```python
from build123d import *

# Parameters (mm, degrees)
SKETCH_1_W          = 206
SKETCH_1_H          = 36
SKETCH_1_W_2        = 200
SKETCH_1_H_2        = 30
EXTRUDE_1_DEPTH     = 20
SKETCH_2_W          = 10
SKETCH_2_H          = 36
EXTRUDE_2_DEPTH     = 4
SKETCH_3_R          = 2.75
CUT_EXTRUDE_1_DEPTH = 4


with BuildPart() as part:
    # 草图1 → 凸台-拉伸1 (new body)
    with BuildSketch(Plane(origin=(0, 0, 0), x_dir=(1, 0, 0), z_dir=(0, 1, 0))):
        Rectangle(SKETCH_1_W, SKETCH_1_H)
        Rectangle(SKETCH_1_W_2, SKETCH_1_H_2, mode=Mode.SUBTRACT)
    extrude(amount=EXTRUDE_1_DEPTH)

    # 草图2 → 凸台-拉伸2 (add)
    with BuildSketch(Plane(origin=(0, 20, 0), x_dir=(1, 0, 0), z_dir=(0, 1, 0))):
        with Locations((-108, 0)):
            Rectangle(SKETCH_2_W, SKETCH_2_H)
        with Locations((108, 0)):
            Rectangle(SKETCH_2_W, SKETCH_2_H)
    extrude(amount=-EXTRUDE_2_DEPTH)

    # 草图3 → 切除-拉伸1 (cut)
    with BuildSketch(Plane(origin=(0, 20, 0), x_dir=(1, 0, 0), z_dir=(0, 1, 0))):
        with Locations(Location((108, 0, 0), (0, 0, 270))):
            Circle(SKETCH_3_R)
        with Locations(Location((-108, 0, 0), (0, 0, 270))):
            Circle(SKETCH_3_R)
    extrude(amount=-CUT_EXTRUDE_1_DEPTH, mode=Mode.SUBTRACT)


solid = part.part
```
Part model, mm, in its own coordinate system. A direction names the side the tool comes from. Coordinates: 2 decimals unless noted, no trailing zeros. Write each loop counter-clockwise with the first axis right and the second up, starting at its lowest first coordinate (ties: lowest second). Pieces come first, ordered by that corner, then holes.
Item 1: Probe line 1 (X direction, y = 17.85, z = 0); line 2 (X direction, y = 13.5, z = -6); line 3 (Z direction, x = -25, y = 12.75). List the from-to ranges inside material, lowest first.
Item 2: Pin check, flat tips, straight feed: pin 1 (3 mm diameter, centred on x = 106.5, z = 9, fed in from -Y); pin 2 (1.5 mm diameter, centred on y = 12, z = -0.5, fed in from +X); pin 3 (4 mm diameter, centred on y = 11, z = 3, fed in from -X). Stop position of each tip, or through.
Item 3: Mould opens along X. For faces 5 (the face through (-100, 10, 0)), 6 (the face through (-113, 18, 0)), 7 (the face through (113, 18, 0)) say: released by +X, released by -X, zero draft, split by the parting line, or undercut.
Item 4: Which spindle directions (+Z, -Z, +X, -X, +Y, -Y) get a long thin tool onto all of the face, cutting with end or side? Do faces 1 (the face through (0, 0, -16)), 2 (the face through (103, 8, 0)), 3 (the face through (-111, 16, 0)), 4 (the face through (-1, 10, -15)). Say none if no direction does.
Item 5: Slice it at A-A (z = 0). Write the cut outline in (x, y).
Item 6: Slice it at D-D (y = 9.75). Write the cut outline in (x, z).
Item 7: Slice it at C-C (x = 108). Write the cut outline in (y, z), and give its area (3 significant figures).
Item 8: Slice it at B-B (z = -11). Write the cut outline in (x, y).
Results found:
1. line 1: x = -113 to -110.75, -105.25 to -100, 100 to 105.25, 110.75 to 113
1. line 2: x = -103 to -100, 100 to 103
1. line 3: z = -18 to -15, 15 to 18
2. pin 1: stops at y = 16
2. pin 2: stops at x = 103
2. pin 3: stops at x = -103
3. face 5: undercut
3. face 6: released by -X
3. face 7: released by +X
4. face 1: +Z, -Z, +X, -X, -Y
4. face 2: +Z, -Z, +X, -Y
4. face 3: +Z, -Z, -X, -Y
4. face 4: +Y, -Y
5. outline: (-113, 16) - (-110.75, 16) - (-110.75, 20) - (-113, 20) - close; (-105.25, 16) - (-103, 16) - (-103, 0) - (-100, 0) - (-100, 20) - (-105.25, 20) - close; (100, 0) - (103, 0) - (103, 16) - (105.25, 16) - (105.25, 20) - (100, 20) - close; (110.75, 16) - (113, 16) - (113, 20) - (110.75, 20) - close
6. outline: (-103, -18) - (103, -18) - (103, 18) - (-103, 18) - close; hole (-100, -15) - (100, -15) - (100, 15) - (-100, 15) - close
7. outline: (16, -18) - (20, -18) - (20, -2.75) - (16, -2.75) - close; (16, 2.75) - (20, 2.75) - (20, 18) - (16, 18) - close
7. area: 122 mm2
8. outline: (-113, 16) - (-103, 16) - (-103, 0) - (-100, 0) - (-100, 20) - (-113, 20) - close; (100, 0) - (103, 0) - (103, 16) - (113, 16) - (113, 20) - (100, 20) - close
